Geometry check sheet. Reference: the model listing, model coordinates, mm. A direction names the side the tool comes from. Round coordinates to 2 decimals unless told otherwise and drop trailing zeros. Order: outer loops, then holes, each group sorted by start corner. A loop starts at its lowest first (then second) coordinate and runs counter-clockwise, first axis right, second up. Notation, with made-up numbers: (-31, -8) - (-27, -8) arc R38 cw to (-27, 31) - close; hole circle Ø5 at (53, 78.25). An arc over 180 degrees is marked (long way). One line per question, with ' | ' between items. Start each with the question number.
Q1. Mould release check, pull along Y, two halves, no side actions. Record for faces 4 (the face through (103.543, 68.481, 12.907)), 5 (the face through (191.2, 88.26, 13.36)), 6 (the face through (104, -38, 6.35)): +Y half, -Y half, draft (parallel to the pull), parting line (faces both ways), or undercut.
Q2. Tool access check on faces 1 (the face through (181.967, 105.775, 3.131)), 2 (the face through (17.844, 85.82, 13.359)), 3 (the face through (178.067, 98.388, 3.131)). Record the directions out of +Z, -Z, +X, -X, +Y, -Y that give a thin tool (end or side, any length) a straight path to the whole face; none if there is none.
Q3. Sectioned sample at A-A, the plane y = 155. Enter the section's corners in (x, z), then the cut area to 3 significant figures.
Q4. Gauge pin test, flat ends, axial feed: P1, Ø1, axis at y = 67.5, z = 8.5, coming from the -X side; P2, Ø3, axis at x = 58.5, z = 9, coming from the -Y side; P3, Ø1, axis at y = 114.5, z = 7, coming from the +X side. Record the tip position at first contact, or that the pin passes through.
Q5. Sectioned sample at C-C, the plane x = 64. Enter the section's corners in (y, z), then the cut area to 3 significant figures.
Q6. Material ranges on line 1 along X through (y, z) = (4, 29.5); line 2 along X through (y, z) = (70, 19); line 3 along Z through (x, y) = (120, 148), recorded low to high.
Q7. Sectioned sample at D-D, the plane y = 42. Enter the section's corners in (x, z).
```python
from build123d import *

# Parameters (mm, degrees)
BOSS_EXTRUDE1_DEPTH     = 209.55
SKETCH1_W               = 240.510539239
SKETCH1_H               = 265.827438106
CUT_EXTRUDE1_DEPTH      = 41.01815501
CUT_EXTRUDE1_DEPTH_BACK = 1
CUT_EXTRUDE2_DEPTH      = 15.875
CUT_EXTRUDE3_DEPTH      = 3.175
SKETCH5_R               = 3
CUT_EXTRUDE4_DEPTH      = 3.175
CUT_EXTRUDE7_DEPTH      = 3.175
CUT_EXTRUDE7_DEPTH_BACK = 6.35
SKETCH7_R               = 2.667
CUT_EXTRUDE8_DEPTH      = 23.690934342
CUT_EXTRUDE9_DEPTH      = 6.35


with BuildPart() as part:
    # Sketch2 → Boss-Extrude1 (new body)
    with BuildSketch(Plane(origin=(0, 0, 0), x_dir=(0, 0, -1), z_dir=(1, 0, 0))):
        Polygon((-19.05, 177.8), (-34.91779298, 0.709477538), (-40.01815501, -56.212476111), (0, -53.790492508), (0, 0), (0, 177.8), align=None)
    extrude(amount=BOSS_EXTRUDE1_DEPTH)

    # Sketch1 → Cut-Extrude1 (cut, two sides)
    with BuildSketch(Plane.XY) as cut_extrude1_sk:
        with Locations((107.411926899, 58.758625739)):
            Rectangle(SKETCH1_W, SKETCH1_H)
        with BuildLine():
            Line((0, 0), (36.195, 174.07688524))
            ThreePointArc((36.195, 174.07688524), (104.775, 149.493461876), (173.355, 174.07688524))
            Line((173.355, 174.07688524), (209.55, 0))
            ThreePointArc((209.55, 0), (104.775, -41.729500882), (0, 0))
        make_face(mode=Mode.SUBTRACT)
    extrude(amount=CUT_EXTRUDE1_DEPTH, mode=Mode.SUBTRACT)
    extrude(cut_extrude1_sk.sketch, amount=-CUT_EXTRUDE1_DEPTH_BACK, mode=Mode.SUBTRACT)

    # Sketch3 → Cut-Extrude2 (cut)
    with BuildSketch(Plane(origin=(0, 3.474785103, 34.670013893), x_dir=(1, 0, 0), z_dir=(0, 0.08924518, 0.996009688))):
        with BuildLine():
            Line((92.029425275, 362.610535175), (16.77359238, -0.776250458))
            ThreePointArc((16.77359238, -0.776250458), (104.775, -31.999740282), (192.77640762, -0.776250458))
            Line((192.77640762, -0.776250458), (117.520574725, 362.610535175))
            Line((117.520574725, 362.610535175), (92.029425275, 362.610535175))
        make_face()
    extrude(amount=-CUT_EXTRUDE2_DEPTH, mode=Mode.SUBTRACT)

    # Sketch4 → Cut-Extrude3 (cut)
    with BuildSketch(Plane(origin=(0, 3.109460703, 34.702747954), x_dir=(1, 0, 0), z_dir=(0, 0.08924518, 0.996009688))):
        Polygon((185.970172739, 112.605103669), (179.585708922, 111.245651158), (183.288614458, 93.855513419), (189.673078275, 95.21496593), align=None)
        Polygon((198.756641777, 51.702635333), (192.545878299, 50.380169071), (196.248783835, 32.990031331), (202.459547313, 34.312497594), align=None)
    extrude(amount=-CUT_EXTRUDE3_DEPTH, mode=Mode.SUBTRACT)

    # Sketch5 → Cut-Extrude4 (cut)
    with BuildSketch(Plane(origin=(0, 3.109460703, 34.702747954), x_dir=(1, 0, 0), z_dir=(0, 0.08924518, 0.996009688))):
        with Locations(Location((25.057058463, 78.729771517, 0), (0, 0, 270))):  # turned: the seam where the file's is
            Circle(SKETCH5_R)
    extrude(amount=-CUT_EXTRUDE4_DEPTH, mode=Mode.SUBTRACT)

    # Sketch6 → Cut-Extrude7 (cut, two sides)
    with BuildSketch(Plane(origin=(0, 0, 0), x_dir=(-1, 0, 0), z_dir=(0, 0, -1))) as cut_extrude7_sk:
        with BuildLine():
            Line((-203.2, -5.683612864), (-203.2, 0.666387136))
            ThreePointArc((-203.2, 0.666387136), (-104.775, -36.938393832), (-6.35, 0.666387136))
            Line((-6.35, 0.666387136), (-6.35, -5.683612864))
            ThreePointArc((-6.35, -5.683612864), (-104.775, -63.961814377), (-203.2, -5.683612864))
        make_face()
    extrude(amount=CUT_EXTRUDE7_DEPTH, mode=Mode.SUBTRACT)
    extrude(cut_extrude7_sk.sketch, amount=-CUT_EXTRUDE7_DEPTH_BACK, mode=Mode.SUBTRACT)

    # Sketch7 → Cut-Extrude8 (cut, through all)
    with BuildSketch(Plane(origin=(0, 1.692693472, 18.891094163), x_dir=(1, 0, 0), z_dir=(0, 0.08924518, 0.996009688))):
        with Locations(Location((104.775, 120.767047718, 0), (0, 0, 270))):  # turned: the seam where the file's is
            Circle(SKETCH7_R)
    extrude(amount=-CUT_EXTRUDE8_DEPTH, mode=Mode.SUBTRACT)

    # Sketch8 → Cut-Extrude9 (cut)
    with BuildSketch(Plane(origin=(0, 0, 0), x_dir=(-1, 0, 0), z_dir=(0, 0, -1))):
        Polygon((-187.325, 106.889315498), (-189.910357143, 94.455252267), (-179.341403396, 92.257698696), (-176.756046253, 104.691761927), align=None)
        Polygon((-32.793953747, 104.691761927), (-22.225, 106.889315498), (-19.639642857, 94.455252267), (-30.208596604, 92.257698696), align=None)
    extrude(amount=-CUT_EXTRUDE9_DEPTH, mode=Mode.SUBTRACT)


solid = part.part
```
Determined:
1) face 4: undercut | face 5: +Y half | face 6: draft
2) face 1: -Z, +X | face 2: +Z, -Z, -X, +Y | face 3: -Z
3) outline: (32.23, 0) - (70.74, 0) - (70.74, 5.15) - (48.73, 5.15) - (48.44, 21.09) - (32.23, 21.09) - close; (138.81, 0) - (177.32, 0) - (177.32, 21.09) - (161.11, 21.09) - (160.82, 5.15) - (138.81, 5.15) - close | area: 918 mm2
4) P1: stops at x = 13.93 | P2: stops at y = -35 | P3: stops at x = 185.85
5) outline: (-36.17, 6.35) - (-31.19, 6.35) - (-31.19, 0) - (157.49, 0) - (157.49, 4.93) - (-23.75, 21.17) - (-22.34, 36.98) - (-36.17, 38.22) - close | area: 2,810 mm2
6) line 1: x = 0.83 to 17.14, 192.41 to 208.72 | line 2: x = 14.55 to 30.95, 178.6 to 195 | line 3: z = 0 to 5.78
7) outline: (8.73, 0) - (200.82, 0) - (200.82, 28.03) - (194.9, 28.03) - (194.96, 31.22) - (184.61, 31.22) - (184.31, 15.28) - (25.24, 15.28) - (24.94, 31.22) - (8.73, 31.22) - close
